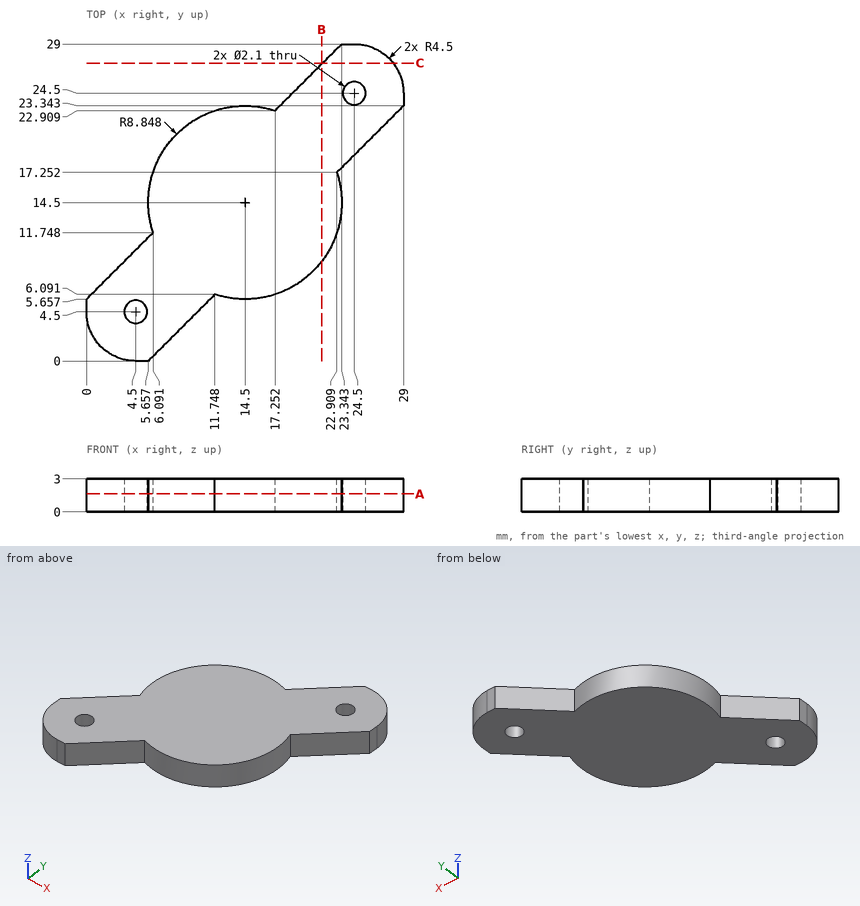
Can you work these out from the drawing? Everything is in mm from the part's minimum corner. Give positions to 0.01 mm unless a question says otherwise; leave off trailing zeros. Loops run counter-clockwise (first coordinate to the right, second up) from the corner with the lowest first, then second, coordinate; pieces in that order, holes last. Notation, with made-up numbers: (34.5, -10) - (84.5, -10) arc R7 ccw to (84.5, 2) - close; hole circle Ø4 at (38.5, 29). An arc over 180 degrees is marked (long way). Use one line per item in the form item = value.
1. I need wall thicknesses on probe 1 along X at (y, z) = (4.25, 0.2) (1 decimal); probe 2 along X at (y, z) = (14.25, 0.85) (1 decimal); probe 3 along X at (y, z) = (11, 2.15) (1 decimal). Which ranges of each line are inside material? Lowest first, please.
Response values:
probe_1 = 0 to 3.5, 5.5 to 9.9
probe_2 = 5.7 to 23.3
probe_3 = 5.3 to 22.6
2. I want a section at A-A (z = 1.65). Please give me the cut outline in (x, y).
Response values:
outline = (0, 4.5) arc R4.5 ccw to (4.5, 0) - (5.66, 0) - (11.75, 6.09) arc R8.85 ccw to (22.91, 17.25) - (29, 23.34) - (29, 24.5) arc R4.5 ccw to (24.5, 29) - (23.34, 29) - (17.25, 22.91) arc R8.85 ccw to (6.09, 11.75) - (0, 5.66) - close; hole circle Ø2.1 at (4.5, 4.5); hole circle Ø2.1 at (24.5, 24.5)
3. I want a section at B-B (x = 21.5). Please give me the cut outline in (y, z), and give its area (3 significant figures).
Response values:
outline = (9.09, 0) - (27.16, 0) - (27.16, 3) - (9.09, 3) - close
area = 54.2 mm²
4. I want a section at C-C (y = 27.25). Please give me the cut outline in (x, z).
Response values:
outline = (21.59, 0) - (28.06, 0) - (28.06, 3) - (21.59, 3) - close
5. I'm going to push flat-ended pins straight in: pin 1 Ø1 at (y, z) = (21.5, 1.5) entering from -X (1 decimal); pin 2 Ø1 at (x, z) = (6.5, 2) entering from +Y (1 decimal). Where does each tip first touch, or does it pass through?
Response values:
pin_1 = 8.5
pin_2 = 19.2
